Part model, mm, in its own coordinate system. A direction names the side the tool comes from. Coordinates: 2 decimals unless noted, no trailing zeros. Answer as CSV lines item,"result".
from build123d import *


with BuildPart() as f1:
    # F0 (on Front) → F1 (revolve)
    with BuildSketch(Plane.XZ):
        with BuildLine():
            Line((15.875, 342.9), (0, 342.9))
            Line((0, 342.9), (0, 328.6125))
            ThreePointArc((0, 328.6125), (1.092488, 311.101104), (4.353008, 293.86128))
            ThreePointArc((4.353008, 293.86128), (5.038673, 291.27063), (5.773488, 288.69349))
            ThreePointArc((5.773488, 288.69349), (30.805227, 252.737075), (72.380527, 238.91875))
            Line((72.380527, 238.91875), (99.4664, 238.91875))
            Line((99.4664, 238.91875), (99.4664, 307.9369))
            Line((99.4664, 307.9369), (89.9414, 307.9369))
            Line((89.9414, 307.9369), (89.9414, 306.3875))
            ThreePointArc((89.9414, 306.3875), (89.476432, 305.264968), (88.3539, 304.8))
            Line((88.3539, 304.8), (67.7164, 304.8))
            ThreePointArc((67.7164, 304.8), (63.226272, 302.940128), (61.3664, 298.45))
            Line((61.3664, 298.45), (61.3664, 289.781537))
            ThreePointArc((61.3664, 289.781537), (49.467276, 274.412476), (31.607907, 282.083209))
            ThreePointArc((31.607907, 282.083209), (19.871918, 311.490581), (15.875, 342.9))
        make_face()
    revolve(axis=Axis((30.470669, 0, 0), (1, 0, 0)))


solid = f1.part
Q1. Two-plate mould, pull along X, no slides. Class faces 3 (the face through (94.637, 300.614, -66.755)), 4 (the face through (61.366, -245, -156)), 5 (the face through (99.466, 181, -158)): released by +X, released by -X, zero draft, split by the parting line, or undercut.
Results:
face 3,"zero draft"
face 4,"undercut"
face 5,"released by +X"
Q2. Wall check: L1, parallel to Z at x = 86, y = 0; L2, parallel to Y at x = 89, z = 0. Give the ranges that are in metal, low to high.
Results:
L1,"z = -304.8 to -238.92, 238.92 to 304.8"
L2,"y = -304.94 to -238.92, 238.92 to 304.94"
Q3. Flat gauge pins, fed straight in: pin 1 (5 mm diameter, centred on y = -155, z = 251.5, fed in from -X); pin 2 (12 mm diameter, centred on y = 272.5, z = 207, fed in from +X); pin 3 (5 mm diameter, centred on y = 274, z = 79, fed in from -X). Where does each tip first touch, or does it go through?
Results:
pin 1,"stops at x = 3.38"
pin 2,"stops at x = 16.05"
pin 3,"stops at x = 6.09"
Q4. Which spindle directions (+Z, -Z, +X, -X, +Y, -Y) get a long thin tool onto all of the face, cutting with end or side? Do faces 1 (the face through (77.891, 185.466, -241.879)), 2 (the face through (0, 176, 278)). Say none if no direction does.
Results:
face 1,"none"
face 2,"+Z, -Z, -X, +Y, -Y"
